Source: CAD feature listing. Evaluate the final solid. Frame: model axes, mm. A direction names the side the tool comes from. Round coordinates to 2 decimals unless told otherwise and drop trailing zeros. Write each loop counter-clockwise with the first axis right and the second up, starting at its lowest first coordinate (ties: lowest second). Pieces come first, ordered by that corner, then holes. Notation, with made-up numbers: M 31,27.25 L 88,27.25 A18 ccw 88,59.25 Z; hole C 86,51 d8. An arc over 180 degrees is marked long. Answer in a Markdown table with one row per item. Add a question column.
Item 1: Mould query, pull axis Z, two halves, no side actions, for faces 4 (the face through (-19, 11.5, -3)), 5 (the face through (-18.99, 6.68, -0.58)), 6 (the face through (-20.993, 5.67, -0.539)). Classes: released by +Z, released by -Z, zero draft, split by the parting line, or undercut.
Item 2: Contact query for flat-ended pins moving along their axis: pin 1 (1 mm diameter, centred on y = 9, z = 8, fed in from -X); pin 2 (1.5 mm diameter, centred on y = 6.5, z = 14.5, fed in from -X); pin 3 (3.5 mm diameter, centred on y = 5, z = -10, fed in from +X). Output: stop coordinate, or through.
Item 3: Cut plane D-D on x = -6.5. Return loops of the section in (y, z).
Item 4: Set-up query: faces 1 (the face through (4.206, 0.493, -4.279)), 2 (the face through (-1, 6, 20)), 3 (the face through (-4, 2, 4)). Return all of +Z, -Z, +X, -X, +Y, -Y with unobstructed straight access to the full face (end or side cutting, diameter ignored); none if empty.
Item 5: Cut plane A-A on x = 0. Return loops of the section in (y, z).
Item 6: Material intervals for probe 1 along Z at (x, y) = (0, 1); probe 2 along X at (y, z) = (2.75, 2.5); probe 3 along X at (y, z) = (5.25, 12), sorted ascending.
Item 7: Cut plane B-B on z = 0. Return loops of the section in (x, y).
Autodesk Inventor part; units mm, degrees
ref_plane "YZ Plane" through (0, 0, 0) normal (1, 0, 0) x (0, 1, 0)
ref_plane "XZ Plane" through (0, 0, 0) normal (0, 1, 0) x (-1, 0, 0)
ref_plane "XY Plane" through (0, 0, 0) normal (0, 0, 1) x (1, 0, 0)
sketch "Sketch9" plane through (0, 0, 0) normal (0, 1, 0) x (-1, 0, 0)
  line L0 (21, 0) -> (-21, 0) construction
  line L1 (0, 21) -> (0, -21) construction
  line L2 (21, -1) -> (20.9762, -1)
  line L3 (21, 1) -> (20.9762, 1)
  line L4 (-20.9762, 1) -> (-21, 1)
  line L5 (1, 21) -> (1, 20.9762)
  line L6 (1, -20.9762) -> (1, -21)
  line L7 (-1, 21) -> (-1, 20.9762)
  line L8 (-1, -5.9161) -> (-1, -21)
  line L9 (-5.9161, -1) -> (-18.9762, -1)
  circle A0 centre (0, 0) radius 5
  arc A1 (-5.9161, -1) -> (-1, -5.9161) centre (0, 0) ccw
  line L10 (-20.9762, -1) -> (-18.9762, -1)
  line L11 (1, -21) -> (1, -3.873) construction
  line L12 (-3.873, 1) -> (-18.9762, 1) construction
  line L13 (-18.9762, 1) -> (-20.9762, 1) construction
  line L14 (-3.873, 1) -> (20.9762, 1) construction
  line L15 (-5.9161, -1) -> (20.9762, -1) construction
  line L16 (1, -3.873) -> (1, 20.9762) construction
  line L17 (-1, -5.9161) -> (-1, 20.9762) construction
  line L18 (0, 21) -> (0, 19) construction
  line L19 (0, 19) -> (1, 19) construction
  arc A2 (-1, -20.9762) -> (0, 21) centre (0, 0) ccw construction
  arc A3 (20.9762, 1) -> (-20.9762, -1) centre (0, 0) ccw construction
  arc A4 (-1, -18.9737) -> (-18.9737, -1) centre (0, 0) ccw
  line L20 (-1, 19) -> (1, 19)
  point P0 (-4.899, -1)
  point P1 (-1, -4.899)
  dimension "d35" = 10
  dimension "d50" = 2
  dimension "d53" = 38
extrude "Extrusion5" add sketch "Sketch9" along normal blind 2
chamfer "Chamfer1" distance 0.5 distance2 1 1 edges at (4.2426, 2, -4.2426) measured on face at (13.5988, 2, 4.219)
sketch "Sketch12" plane through (0, 0, 0) normal (0, 1, 0) x (-1, 0, 0)
  circle A0 centre (0, 0) radius 5
  line L0 (-18.9737, -1) -> (-5.9161, -1)
  line L1 (-18.9737, -1) -> (-20.9762, -1)
  line L2 (-1, -5.9161) -> (-1, -18.9737)
  line L3 (-1, -18.9737) -> (-1, -20.9762)
  line L4 (-1, -20.9762) -> (-1, 20.9762) construction
  line L5 (-20.9762, -1) -> (20.9762, -1) construction
  line L6 (1, -20.9762) -> (1, 20.9762) construction
  line L7 (-20.9762, 1) -> (20.9762, 1) construction
  line L8 (-1, 20.9762) -> (-1, 18.9762)
  line L9 (1, 20.9762) -> (1, 18.9762)
  arc A1 (-1, -20.9762) -> (1, 20.9762) centre (0, 0) ccw
  arc A2 (-1, 20.9762) -> (-20.9762, -1) centre (0, 0) ccw
  line L10 (-1, -18) -> (-1, -20.9762)
  line L11 (-17.9722, -1) -> (-20.9762, -1)
  line L12 (1, 20.9762) -> (1, 18.9737)
  line L13 (-1, 20.9762) -> (-1, 18.9737)
  arc A3 (-1, -18.9737) -> (1, 18.9737) centre (0, 0) ccw
  arc A4 (-1, 18.9737) -> (-18.9737, -1) centre (0, 0) ccw
  line L14 (1, 18.9762) -> (0.9512, 18.9762)
  line L15 (-0.9512, 18.9762) -> (-1, 18.9762)
  line L16 (1, 18.9762) -> (0.9512, 18.9762)
  line L17 (-0.9512, 18.9762) -> (-1, 18.9762)
  point P0 (-5.4083, -1)
  point P1 (-1, -5.4083)
  point P2 (-1, 17.9722)
  point P3 (1, 18.9737)
  dimension "d63" = 2
  dimension "d64" = 2
  dimension "d65" = 2
  dimension "d66" = 2
extrude "Extrusion8" add sketch "Sketch12" along normal blind 11.5 contours L1 A2 L8 L13 A4 | A3 L12 L9 A1 L3
properties part number "base layer 2"
Results below:
| question | item | result |
|---|---|---|
| 1 | face 4 | zero draft |
| 1 | face 5 | undercut |
| 1 | face 6 | split by the parting line |
| 2 | pin 1 | x = -19.62 |
| 2 | pin 2 | x = -15.87 |
| 2 | pin 3 | x = -14.93 |
| 3 | outline | M 0,-19.97 L 11.5,-19.97 L 11.5,-17.85 L 2,-17.85 L 2,17.85 L 11.5,17.85 L 11.5,19.97 L 0,19.97 Z |
| 4 | face 1 | -Z, +X, +Y, -Y |
| 4 | face 2 | +Z, +Y, -Y |
| 4 | face 3 | +Y |
| 5 | outline | M 0,-21 L 11.5,-21 L 11.5,-19 L 2,-19 L 2,-5 L 0,-5 Z; M 0,5 L 2,5 L 2,19 L 0,19 Z |
| 6 | probe 1 | -21 to -5, 5 to 19 |
| 6 | probe 2 | -20.85 to -18.83, 18.83 to 20.85 |
| 6 | probe 3 | -17.23 to -14.73, 14.73 to 17.23 |
| 7 | outline | M -21,0 L -5,0 L -5,2 L -19,2 L -19,11.5 L -21,11.5 Z; M 5,0 L 21,0 L 21,11.5 L 19,11.5 L 19,2 L 5,2 Z |
